```python
from build123d import *

# Parameters (mm, degrees)
SKETCH2_W           = 10
SKETCH2_H           = 18
SKETCH2_R           = 2
BOSS_EXTRUDE1_DEPTH = 5
SKETCH3_W           = 30
SKETCH3_H           = 30
BOSS_EXTRUDE2_DEPTH = 5
FILLET1_R           = 5
FILLET2_R           = 3
SKETCH4_R           = 2
CUT_EXTRUDE1_DEPTH  = 5


with BuildPart() as part:
    # Sketch2 → Boss-Extrude1 (new body)
    with BuildSketch(Plane.XY):
        with Locations((-5, 9)):
            Rectangle(SKETCH2_W, SKETCH2_H)
        with Locations((-5, 4.24)):
            Circle(SKETCH2_R, mode=Mode.SUBTRACT)
    extrude(amount=BOSS_EXTRUDE1_DEPTH)

    # Sketch3 → Boss-Extrude2 (add)
    with BuildSketch(Plane(origin=(0, 18, 0), x_dir=(1, 0, 0), z_dir=(0, 1, 0))):
        with Locations((-5, -2.5)):
            Rectangle(SKETCH3_W, SKETCH3_H)
    extrude(amount=-BOSS_EXTRUDE2_DEPTH)

    # Fillet1
    fillet1_edges = [part.edges().sort_by_distance(p)[0] for p in [
        (0, 13, 2.5),
        (-10, 13, 2.5),
    ]]
    fillet(fillet1_edges, radius=FILLET1_R)

    # Fillet2
    fillet2_edges = [part.edges().sort_by_distance(p)[0] for p in [
        (0, 0, 2.5),
        (-10, 0, 2.5),
    ]]
    fillet(fillet2_edges, radius=FILLET2_R)

    # Sketch4 → Cut-Extrude1 (cut)
    with BuildSketch(Plane(origin=(0, 18, 0), x_dir=(1, 0, 0), z_dir=(0, 1, 0))):
        with Locations(Location((-16, 8.5, 0), (0, 0, 270))):
            Circle(SKETCH4_R)
        with Locations(Location((6, 8.5, 0), (0, 0, 270))):
            Circle(SKETCH4_R)
        with Locations(Location((6, -13.5, 0), (0, 0, 270))):
            Circle(SKETCH4_R)
        with Locations(Location((-16, -13.5, 0), (0, 0, 270))):
            Circle(SKETCH4_R)
    extrude(amount=-CUT_EXTRUDE1_DEPTH, mode=Mode.SUBTRACT)


solid = part.part
```
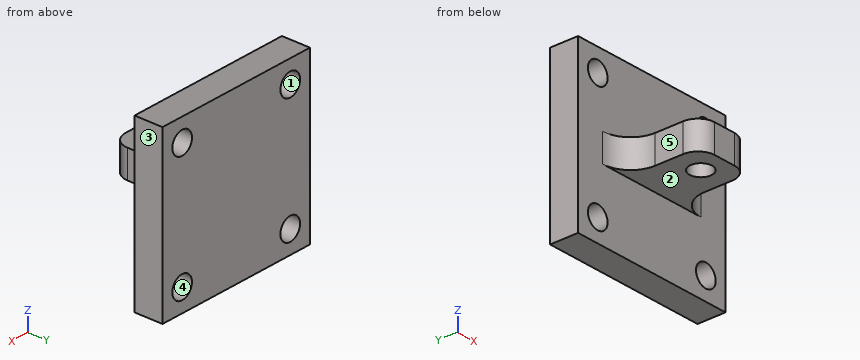
Can you work these out from the model? Positions are in its coordinate system, mm. Face numbers are marked on the shaded views. A direction names the side the tool comes from. Coordinates: 2 decimals unless noted, no trailing zeros. Loops run counter-clockwise (first coordinate to the right, second up) from the corner with the lowest first, then second, coordinate; pieces in that order, holes last.
Item 1: I'm going to push flat-ended pins straight in: pin 1 (1.5 mm diameter, centred on y = 4.5, z = 1.5, fed in from +X); pin 2 (3 mm diameter, centred on x = 6, z = 13.5, fed in from -Y); pin 3 (1.5 mm diameter, centred on x = -4, y = 7, fed in from +Z); pin 4 (5 mm diameter, centred on x = -5, y = 4.24, fed in from -Z). Where does each tip first touch, or does it pass through?
Answers below:
pin 1: stops at x = 0
pin 2: passes through
pin 3: stops at z = 5
pin 4: stops at z = 0
Item 2: Suppose I cut it at D-D (x = -5). Please give me the cut outline in (y, z), then the cut area to 3 significant figures.
Answers below:
outline: (0, 0) - (2.24, 0) - (2.24, 5) - (0, 5) - close; (6.24, 0) - (13, 0) - (13, -12.5) - (18, -12.5) - (18, 17.5) - (13, 17.5) - (13, 5) - (6.24, 5) - close
area: 195 mm2
Item 3: Suppose I cut it at A-A (x = 6). Please give me the cut outline in (y, z), then the cut area to 3 significant figures.
Answers below:
outline: (13, -12.5) - (18, -12.5) - (18, -10.5) - (13, -10.5) - close; (13, -6.5) - (18, -6.5) - (18, 11.5) - (13, 11.5) - close; (13, 15.5) - (18, 15.5) - (18, 17.5) - (13, 17.5) - close
area: 110 mm2
Item 4: Please list where these lines run through material, in increasing order: L1, parallel to X at y = 14, z = -8.5; L2, parallel to X at y = 14, z = 12; L3, parallel to Y at x = -5, z = 3.75.
Answers below:
L1: x = -20 to -18, -14 to 4, 8 to 10
L2: x = -20 to -17.32, -14.68 to 4.68, 7.32 to 10
L3: y = 0 to 2.24, 6.24 to 18
Item 5: Which directions (+Z, -Z, +X, -X, +Y, -Y) give clear straight access to the entire face, cutting with the end or side of a thin tool? Please do the marked faces 4 and 5.
Answers below:
face 4: +Y, -Y
face 5: +Z, -Z, -X, -Y
Item 6: Suppose I cut it at B-B (z = -8.5). Please give me the cut outline in (x, y).
Answers below:
outline: (-20, 13) - (-18, 13) - (-18, 18) - (-20, 18) - close; (-14, 13) - (4, 13) - (4, 18) - (-14, 18) - close; (8, 13) - (10, 13) - (10, 18) - (8, 18) - close
Item 7: Suppose I cut it at C-C (y = 4.24). Please give me the cut outline in (x, z), then the cut area to 3 significant figures.
Answers below:
outline: (-10, 0) - (-7, 0) - (-7, 5) - (-10, 5) - close; (-3, 0) - (0, 0) - (0, 5) - (-3, 5) - close
area: 30.0 mm2
Item 8: If we mould it in two halves opening along Z, with no side actions, what happens to the marked faces 1, 2 and 3? For each: released by +Z, released by -Z, zero draft, split by the parting line, or undercut.
Answers below:
face 1: undercut
face 2: released by -Z
face 3: zero draft
